Part model, mm, in its own coordinate system. A direction names the side the tool comes from. Give positions to 0.01 mm unless a question says otherwise; leave off trailing zeros. Order: outer loops, then holes, each group sorted by start corner. A loop starts at its lowest first (then second) coordinate and runs counter-clockwise, first axis right, second up. Notation, with made-up numbers: (26.5, 36) - (76.5, 36) arc R6 ccw to (76.5, 42) - close; hole circle Ø8 at (78.5, 21). An arc over 180 degrees is marked (long way). Use one line per item in the form item = value. Start each with the question number.
1. Band-saw the part on D-D, the plane y = 4. List the corners of the cut face in (x, z).
2. Pull direction Z, two halves, no side cores. Call faces 4 (the face through (3.2, 5.7, -0.6)), 5 (the face through (3, 1, 0.6)), 6 (the face through (3.65, 1.3, 0.3)): +Z half, -Z half, draft (parallel to the pull), parting line (faces both ways), or undercut.
3. Band-saw the part on A-A, the plane x = 1.5. List the corners of the cut face in (y, z).
4. Drill centre lines: line 1 (Y direction, x = 4.25, z = -0.85); line 2 (X direction, y = 3.15, z = -0.3); line 3 (X direction, y = 4.35, z = -0.4). Where is each one in solid material? Low to high.
5. Tool access for faces 1 (the face through (3.2, 3.8, -0.6)), 2 (the face through (3, 5, 0.6)), 3 (the face through (3.315, 4.504, 0.296)): list every direction of +Z, -Z, +X, -X, +Y, -Y with a clear straight run to the whole face (end or side of a thin tool).
6. Band-saw the part on B-B, the plane y = 5.3. List the corners of the cut face in (x, z).
7. Band-saw the part on C-C, the plane y = 2.85. List the corners of the cut face in (x, z), plus the area to 3 significant figures.
8. Pin check, flat tip, straight feed: P1, Ø0.8, axis at x = 5.5, y = 3, coming from the +Z side. Stop position of the tip, or through.
from build123d import *

# Parameters (mm, degrees)
SKETCH1_W           = 6.5
SKETCH1_H           = 1.27
BOSS_EXTRUDE1_DEPTH = 0.3
BOSS_EXTRUDE2_DEPTH = 1.6
BOSS_EXTRUDE3_START = 1.9
SKETCH1_2_W         = 6.5
SKETCH1_2_H         = 1.27
BOSS_EXTRUDE3_DEPTH = 0.3
BOSS_EXTRUDE4_START = 1.9
BOSS_EXTRUDE4_DEPTH = 1.6
BOSS_EXTRUDE5_START = 3.8
SKETCH1_3_W         = 6.5
SKETCH1_3_H         = 1.27
BOSS_EXTRUDE5_DEPTH = 0.3
BOSS_EXTRUDE6_START = 3.8
BOSS_EXTRUDE6_DEPTH = 1.6
BOSS_EXTRUDE7_START = 5.7
SKETCH1_4_W         = 6.5
SKETCH1_4_H         = 1.27
BOSS_EXTRUDE7_DEPTH = 0.3
SKETCH3_W           = 4
SKETCH3_H           = 5.4
BOSS_EXTRUDE8_DEPTH = 0.2
SKETCH4_R           = 0.5
BOSS_EXTRUDE9_DEPTH = 0.6


with BuildPart() as part:
    # Sketch1 → Boss-Extrude1 (new body)
    with BuildSketch(Plane(origin=(0, 0, 0), x_dir=(1, 0, 0), z_dir=(0, 1, 0))):
        with Locations((3.25, 0.635)):
            Rectangle(SKETCH1_W, SKETCH1_H)
    extrude(amount=BOSS_EXTRUDE1_DEPTH)

    # Sketch2 → Boss-Extrude2 (add)
    with BuildSketch(Plane(origin=(0, 0.3, 0), x_dir=(1, 0, 0), z_dir=(0, 1, 0))):
        with BuildLine():
            Line((1.25, 0.2), (0.5, 0.2))
            ThreePointArc((0.5, 0.2), (0.287867966, 0.287867966), (0.2, 0.5))
            Line((0.2, 0.5), (0.2, 0.77))
            ThreePointArc((0.2, 0.77), (0.287867966, 0.982132034), (0.5, 1.07))
            Line((0.5, 1.07), (6, 1.07))
            ThreePointArc((6, 1.07), (6.212132034, 0.982132034), (6.3, 0.77))
            Line((6.3, 0.77), (6.3, 0.5))
            ThreePointArc((6.3, 0.5), (6.212132034, 0.287867966), (6, 0.2))
            Line((6, 0.2), (5.25, 0.2))
            Line((5.25, 0.2), (5.25, 0.05))
            Line((5.25, 0.05), (6, 0.05))
            ThreePointArc((6, 0.05), (6.318198052, 0.181801948), (6.45, 0.5))
            Line((6.45, 0.5), (6.45, 0.77))
            ThreePointArc((6.45, 0.77), (6.318198052, 1.088198052), (6, 1.22))
            Line((6, 1.22), (0.5, 1.22))
            ThreePointArc((0.5, 1.22), (0.181801948, 1.088198052), (0.05, 0.77))
            Line((0.05, 0.77), (0.05, 0.5))
            ThreePointArc((0.05, 0.5), (0.181801948, 0.181801948), (0.5, 0.05))
            Line((0.5, 0.05), (1.25, 0.05))
            Line((1.25, 0.05), (1.25, 0.2))
        make_face()
    extrude(amount=BOSS_EXTRUDE2_DEPTH)

    # Sketch1<2> → Boss-Extrude3 (add)
    with BuildSketch(Plane(origin=(0, 0, 0), x_dir=(1, 0, 0), z_dir=(0, 1, 0)).offset(BOSS_EXTRUDE3_START)):
        with Locations((3.25, 0.635)):
            Rectangle(SKETCH1_2_W, SKETCH1_2_H)
    extrude(amount=BOSS_EXTRUDE3_DEPTH)

    # Sketch2<3> → Boss-Extrude4 (add)
    with BuildSketch(Plane(origin=(0, 0.3, 0), x_dir=(1, 0, 0), z_dir=(0, 1, 0)).offset(BOSS_EXTRUDE4_START)):
        with BuildLine():
            Line((1.25, 0.2), (0.5, 0.2))
            ThreePointArc((0.5, 0.2), (0.287867966, 0.287867966), (0.2, 0.5))
            Line((0.2, 0.5), (0.2, 0.77))
            ThreePointArc((0.2, 0.77), (0.287867966, 0.982132034), (0.5, 1.07))
            Line((0.5, 1.07), (6, 1.07))
            ThreePointArc((6, 1.07), (6.212132034, 0.982132034), (6.3, 0.77))
            Line((6.3, 0.77), (6.3, 0.5))
            ThreePointArc((6.3, 0.5), (6.212132034, 0.287867966), (6, 0.2))
            Line((6, 0.2), (5.25, 0.2))
            Line((5.25, 0.2), (5.25, 0.05))
            Line((5.25, 0.05), (6, 0.05))
            ThreePointArc((6, 0.05), (6.318198052, 0.181801948), (6.45, 0.5))
            Line((6.45, 0.5), (6.45, 0.77))
            ThreePointArc((6.45, 0.77), (6.318198052, 1.088198052), (6, 1.22))
            Line((6, 1.22), (0.5, 1.22))
            ThreePointArc((0.5, 1.22), (0.181801948, 1.088198052), (0.05, 0.77))
            Line((0.05, 0.77), (0.05, 0.5))
            ThreePointArc((0.05, 0.5), (0.181801948, 0.181801948), (0.5, 0.05))
            Line((0.5, 0.05), (1.25, 0.05))
            Line((1.25, 0.05), (1.25, 0.2))
        make_face()
    extrude(amount=BOSS_EXTRUDE4_DEPTH)

    # Sketch1<3> → Boss-Extrude5 (add)
    with BuildSketch(Plane(origin=(0, 0, 0), x_dir=(1, 0, 0), z_dir=(0, 1, 0)).offset(BOSS_EXTRUDE5_START)):
        with Locations((3.25, 0.635)):
            Rectangle(SKETCH1_3_W, SKETCH1_3_H)
    extrude(amount=BOSS_EXTRUDE5_DEPTH)

    # Sketch2<4> → Boss-Extrude6 (add)
    with BuildSketch(Plane(origin=(0, 0.3, 0), x_dir=(1, 0, 0), z_dir=(0, 1, 0)).offset(BOSS_EXTRUDE6_START)):
        with BuildLine():
            Line((1.25, 0.2), (0.5, 0.2))
            ThreePointArc((0.5, 0.2), (0.287867966, 0.287867966), (0.2, 0.5))
            Line((0.2, 0.5), (0.2, 0.77))
            ThreePointArc((0.2, 0.77), (0.287867966, 0.982132034), (0.5, 1.07))
            Line((0.5, 1.07), (6, 1.07))
            ThreePointArc((6, 1.07), (6.212132034, 0.982132034), (6.3, 0.77))
            Line((6.3, 0.77), (6.3, 0.5))
            ThreePointArc((6.3, 0.5), (6.212132034, 0.287867966), (6, 0.2))
            Line((6, 0.2), (5.25, 0.2))
            Line((5.25, 0.2), (5.25, 0.05))
            Line((5.25, 0.05), (6, 0.05))
            ThreePointArc((6, 0.05), (6.318198052, 0.181801948), (6.45, 0.5))
            Line((6.45, 0.5), (6.45, 0.77))
            ThreePointArc((6.45, 0.77), (6.318198052, 1.088198052), (6, 1.22))
            Line((6, 1.22), (0.5, 1.22))
            ThreePointArc((0.5, 1.22), (0.181801948, 1.088198052), (0.05, 0.77))
            Line((0.05, 0.77), (0.05, 0.5))
            ThreePointArc((0.05, 0.5), (0.181801948, 0.181801948), (0.5, 0.05))
            Line((0.5, 0.05), (1.25, 0.05))
            Line((1.25, 0.05), (1.25, 0.2))
        make_face()
    extrude(amount=BOSS_EXTRUDE6_DEPTH)

    # Sketch1<4> → Boss-Extrude7 (add)
    with BuildSketch(Plane(origin=(0, 0, 0), x_dir=(1, 0, 0), z_dir=(0, 1, 0)).offset(BOSS_EXTRUDE7_START)):
        with Locations((3.25, 0.635)):
            Rectangle(SKETCH1_4_W, SKETCH1_4_H)
    extrude(amount=BOSS_EXTRUDE7_DEPTH)

    # Sketch3 → Boss-Extrude8 (add)
    with BuildSketch(Plane.XY):
        with Locations((3.25, 3)):
            Rectangle(SKETCH3_W, SKETCH3_H)
    extrude(amount=-BOSS_EXTRUDE8_DEPTH)

    # Sketch4 → Boss-Extrude9 (add)
    with BuildSketch(Plane.XY):
        with Locations(Location((3.25, 5, 0), (0, 0, 180))):
            Circle(SKETCH4_R)
        with Locations(Location((3.25, 1, 0), (0, 0, 180))):
            Circle(SKETCH4_R)
    extrude(amount=BOSS_EXTRUDE9_DEPTH)


solid = part.part
From the geometry:
q1.outline = (0, -1.27) - (6.5, -1.27) - (6.5, 0) - (0, 0) - close
q2.face_4 = undercut
q2.face_5 = +Z half
q2.face_6 = draft
q3.outline = (0, -1.27) - (0.3, -1.27) - (0.3, -1.22) - (1.9, -1.22) - (1.9, -1.27) - (2.2, -1.27) - (2.2, -1.22) - (3.8, -1.22) - (3.8, -1.27) - (4.1, -1.27) - (4.1, -1.22) - (5.7, -1.22) - (5.7, -1.27) - (6, -1.27) - (6, 0) - (0, 0) - close; hole (0.3, -1.07) - (1.9, -1.07) - (1.9, -0.2) - (0.3, -0.2) - close; hole (2.2, -1.07) - (3.8, -1.07) - (3.8, -0.2) - (2.2, -0.2) - close; hole (4.1, -1.07) - (5.7, -1.07) - (5.7, -0.2) - (4.1, -0.2) - close
q4.line_1 = 0 to 0.3, 1.9 to 2.2, 3.8 to 4.1, 5.7 to 6
q4.line_2 = 0.1 to 0.28, 6.22 to 6.4
q4.line_3 = 0.06 to 0.22, 6.28 to 6.44
q5.face_1 = none
q5.face_2 = +Z, +X, -X, +Y, -Y
q5.face_3 = +Z
q6.outline = (0.05, -0.77) arc R0.45 ccw to (0.5, -1.22) - (6, -1.22) arc R0.45 ccw to (6.45, -0.77) - (6.45, -0.5) arc R0.45 ccw to (6, -0.05) - (5.25, -0.05) - (5.25, 0) - (3.65, 0) - (3.65, 0.6) - (2.85, 0.6) - (2.85, 0) - (1.25, 0) - (1.25, -0.05) - (0.5, -0.05) arc R0.45 ccw to (0.05, -0.5) - close; hole (0.2, -0.77) arc R0.3 ccw to (0.5, -1.07) - (6, -1.07) arc R0.3 ccw to (6.3, -0.77) - (6.3, -0.5) arc R0.3 ccw to (6, -0.2) - (0.5, -0.2) arc R0.3 ccw to (0.2, -0.5) - close
q7.outline = (0.05, -0.77) arc R0.45 ccw to (0.5, -1.22) - (6, -1.22) arc R0.45 ccw to (6.45, -0.77) - (6.45, -0.5) arc R0.45 ccw to (6, -0.05) - (5.25, -0.05) - (5.25, 0) - (1.25, 0) - (1.25, -0.05) - (0.5, -0.05) arc R0.45 ccw to (0.05, -0.5) - close; hole (0.2, -0.77) arc R0.3 ccw to (0.5, -1.07) - (6, -1.07) arc R0.3 ccw to (6.3, -0.77) - (6.3, -0.5) arc R0.3 ccw to (6, -0.2) - (0.5, -0.2) arc R0.3 ccw to (0.2, -0.5) - close
q7.area = 2.28 mm²
q8.P1 = 0
